from build123d import *

# Parameters (mm, degrees)
SKETCH063_W            = 78
SKETCH063_H            = 18
PAD020_DEPTH           = 3
SKETCH064_R            = 5.25
POCKET040_DEPTH        = 2
LINEARPATTERN001_COUNT = 2
LINEARPATTERN001_PITCH = 66
SKETCH065_W            = 35
SKETCH065_H            = 18
PAD021_DEPTH           = 86
SKETCH066_R            = 7.75
POCKET041_DEPTH        = 83
POCKET042_DEPTH        = 3
SKETCH068_W            = 20
SKETCH068_H            = 36
POCKET043_DEPTH        = 18.001
SKETCH069_R            = 10
POCKET044_DEPTH        = 18.001
FILLET_R               = 1


with BuildPart() as part:
    # Sketch063 → Pad020 (new body)
    with BuildSketch(Plane.XY):
        with Locations((0, 29.5)):
            Rectangle(SKETCH063_W, SKETCH063_H)
    extrude(amount=PAD020_DEPTH)

    # Sketch064 (on Face6 of Pad020) → Pocket040 (cut)
    with BuildSketch(Plane.XY.offset(3)):
        with Locations((-33, 29.5)):
            Circle(SKETCH064_R)
    pocket040 = extrude(amount=-POCKET040_DEPTH, mode=Mode.SUBTRACT)

    # LinearPattern001: Pocket040 ×2
    with Locations(*[(i * LINEARPATTERN001_PITCH, 0, 0) for i in range(1, LINEARPATTERN001_COUNT)]):
        add(pocket040, mode=Mode.SUBTRACT)

    # Sketch065 (on Face5 of LinearPattern001) → Pad021 (join)
    with BuildSketch(Plane.XY.offset(3)):
        with Locations((0, 29.5)):
            Rectangle(SKETCH065_W, SKETCH065_H)
    extrude(amount=PAD021_DEPTH)

    # Sketch066 (on Face12 of Pad021) → Pocket041 (cut)
    with BuildSketch(Plane.XY.offset(89)):
        with Locations((0, 29.5)):
            Circle(SKETCH066_R)
    extrude(amount=-POCKET041_DEPTH, mode=Mode.SUBTRACT)

    # Sketch067 (on Face12 of Pocket041) → Pocket042 (cut)
    with BuildSketch(Plane.XY.offset(89)):
        Polygon((-10.25, 38.5), (10.25, 38.5), (14.25, 35.5), (14.25, 23.5), (10.25, 20.5), (-10.25, 20.5), (-14.25, 23.5), (-14.25, 35.5), align=None)
    extrude(amount=-POCKET042_DEPTH, mode=Mode.SUBTRACT)

    # Sketch068 (on Face6 of Pocket042) → Pocket043 (cut, through all)
    with BuildSketch(Plane(origin=(0, 38.5, 0), x_dir=(-1, 0, 0), z_dir=(0, 1, 0))):
        with Locations((0, 27)):
            Rectangle(SKETCH068_W, SKETCH068_H)
    extrude(amount=-POCKET043_DEPTH, mode=Mode.SUBTRACT)

    # Sketch069 (on Face22 of Pocket043) → Pocket044 (cut, through all)
    with BuildSketch(Plane.XZ.offset(-20.5)):
        with Locations((0, 45)):
            Circle(SKETCH069_R)
    extrude(amount=-POCKET044_DEPTH, mode=Mode.SUBTRACT)

    # Fillet
    fillet_edges = [part.edges().sort_by_distance(p)[0] for p in [
        (-7.75, 29.5, 9),
        (7.75, 29.5, 7.5),
        (-7.75, 29.5, 6),
    ]]
    fillet(fillet_edges, radius=FILLET_R)


with BuildPart() as part_1:
    # Body005 placement: moved
    add(part.part.moved(Location((0, 0, 32))))


solid = part_1.part
Build history of the part. All positions in model axes, mm. A direction names the side the tool comes from. Round coordinates to 2 decimals unless told otherwise and drop trailing zeros. Write each loop counter-clockwise with the first axis right and the second up, starting at its lowest first coordinate (ties: lowest second). Pieces come first, ordered by that corner, then holes. Notation, with made-up numbers: M 58.25,-5.75 L 108.25,-5.75 A13 ccw 108.25,3.25 Z; hole C 34.25,-5 d3. An arc over 180 degrees is marked long. Answer as a JSON object with one key per item and string values. Group by question number.
(1) Cut at B-B (x = 0). Give the cut face in (y, z), and give its area (3 significant figures).
(2) Mould opens along Z. For faces 1 (the flat face through (2.3, 20.9, 41)), 2 (the flat face through (15, 30, 121)), 3 (the flat face through (12.278, 22.021, 119.521)) say: pulls with the +Z half, pulls with the -Z half, needs draft (parallel to the pull), parting line crosses it, or undercut.
(3) Cut at C-C (z = 110). Give the cut face in (x, y), and give its area (3 significant figures).
(4) Cut at A-A (z = 49.5). Give the cut face in (x, y).
(5) Which spindle directions (+Z, -Z, +X, -X, +Y, -Y) get a long thin tool onto all of the face, cutting with end or side? Do faces 4 (the flat face through (-12.28, 36.98, 119.52)), 5 (the flat face through (11, 20.5, 73)), 6 (the cylindrical face through (8.768, 29.374, 81.808)), 7 (the flat face through (26, 30, 35)), 8 (the flat face through (-39, 29, 33)). Say none if no direction does.
(6) Cut at D-D (x = -33). Give the cut face in (y, z).
(7) Flat gauge pins, fed straight in: pin 1 (9 mm diameter, centred on x = -27.5, y = 26.5, fed in from +Z); pin 2 (3.5 mm diameter, centred on y = 30.5, z = 119.5, fed in from -X); pin 3 (0.9 mm diameter, centred on y = 27, z = 120, fed in from +X). Where does each tip first touch, or does it go through?
(8) Drill centre lines: L1, parallel to X at y = 28, z = 51; L2, parallel to X at y = 29.5, z = 105; L3, parallel to Y at x = 0, z = 92. Where is each one in solid material? Low to high.
Responses:
{
 "1": {"outline": "M 20.5,32 L 38.5,32 L 38.5,41 L 38.25,41 A1 ccw 37.25,40 L 37.25,39 A1 cw 36.25,38 L 22.75,38 A1 cw 21.75,39 L 21.75,40 A1 ccw 20.75,41 L 20.5,41 Z; M 20.5,87 L 21.75,87 L 21.75,118 L 20.5,118 Z; M 37.25,87 L 38.5,87 L 38.5,118 L 37.25,118 Z", "area": "193 mm2"},
 "2": {"face 1": "undercut", "face 2": "pulls with the +Z half", "face 3": "needs draft"},
 "3": {"outline": "M -17.5,20.5 L 17.5,20.5 L 17.5,38.5 L -17.5,38.5 Z; hole C 0,29.5 d15.5", "area": "441 mm2"},
 "4": {"outline": "M -17.5,20.5 L -10,20.5 L -10,38.5 L -17.5,38.5 Z; M 10,20.5 L 17.5,20.5 L 17.5,38.5 L 10,38.5 Z"},
 "5": {"face 4": "+Z", "face 5": "+Z, -Z, +X, -X, -Y", "face 6": "+Y, -Y", "face 7": "+Z, +X, +Y, -Y", "face 8": "+Z, -Z, -X, +Y, -Y"},
 "6": {"outline": "M 20.5,32 L 38.5,32 L 38.5,35 L 34.75,35 L 34.75,33 L 24.25,33 L 24.25,35 L 20.5,35 Z"},
 "7": {"pin 1": "stops at z = 35", "pin 2": "stops at x = -17.5", "pin 3": "stops at x = 17.5"},
 "8": {"L1": "x = -17.5 to -10, 10 to 17.5", "L2": "x = -17.5 to -7.75, 7.75 to 17.5", "L3": "y = 20.5 to 21.75, 37.25 to 38.5"}
}
